For this review, take the finished solid that the model builds, in its own axes (mm). A direction names the side the tool comes from. Round coordinates to 2 decimals unless told otherwise and drop trailing zeros. Loops run counter-clockwise (first coordinate to the right, second up) from the corner with the lowest first, then second, coordinate; pieces in that order, holes last. Notation, with made-up numbers: M -31.75,6.25 L 12.25,6.25 A13 ccw 12.25,24.25 Z; hole C 25,65.25 d7. An arc over 180 degrees is marked long. One line per question, with ' | ' between items. Start each with the question number.
1) For pin 1 Ø3.5 at (x, z) = (49, 57.5) entering from +Y; pin 2 Ø0.9 at (x, z) = (-49, 57.5) entering from -Y; pin 3 Ø0.9 at (x, y) = (49, -1) entering from +Z, all flat-tipped, find the tip position at first contact; note any pin that passes through.
2) Mouldability with a two-part tool opening along X and no side actions: class faces 5 (the face through (-49, 29, 30)), 6 (the face through (47, 0, 30)), 7 (the face through (-48, -5, 58)) as pulls with the +X half, pulls with the -X half, needs draft (parallel to the pull), parting line crosses it, or undercut.
3) We need section D-D (z = 47.5). Give the boundary of the cut face in (x, y), and give its area (3 significant figures).
4) We need section B-B (y = 2). Give the boundary of the cut face in (x, z).
5) For probe 1 along Y at (x, z) = (-37, 19); probe 2 along X at (y, z) = (-3, 14.5); probe 3 along X at (y, z) = (26.5, 24), list the stretches that pass through material, from the lowest coordinate up. Write a range as from..to.
6) For faces 1 (the face through (-3, 30, 0)), 2 (the face through (-1, 28, 30)), 3 (the face through (49, 5, 58)), 4 (the face through (25, -30, 26)), list the 3-axis set-ups (+Z, -Z, +X, -X, +Y, -Y) from which the entire face can be reached by the end or side of a thin tool; tool diameter is ignored.
7) We need section A-A (x = -33.5). Give the boundary of the cut face in (y, z), and give its area (3 significant figures).
8) We need section C-C (x = 25). Give the boundary of the cut face in (y, z), and give its area (3 significant figures).
```python
from build123d import *

# Parameters (mm, degrees)
EXTRUDE_1_DEPTH          = 60
EXTRUDE_2_DEPTH          = 60
SKETCH_4_R               = 1.4
CUT_EXTRUDE_1_DEPTH      = 60
MIRROR_2_COPY_1_DEPTH    = 60
MIRROR_2_COPY_2_SKETCH_R = 1.4
MIRROR_2_COPY_2_DEPTH    = 60
SKETCH_7_R               = 6
CUT_EXTRUDE_3_DEPTH      = 10
SKETCH_8_W               = 4
SKETCH_8_H               = 10
CUT_EXTRUDE_4_DEPTH      = 100


with BuildPart() as part:
    # 草图1 → 凸台-拉伸1 (new body)
    with BuildSketch(Plane.XY):
        with BuildLine():
            Line((-45, 31), (45, 31))
            ThreePointArc((45, 31), (48.535533906, 29.535533906), (50, 26))
            Line((50, 26), (50, -26))
            ThreePointArc((50, -26), (48.535533906, -29.535533906), (45, -31))
            Line((45, -31), (-45, -31))
            ThreePointArc((-45, -31), (-48.535533906, -29.535533906), (-50, -26))
            Line((-50, -26), (-50, 26))
            ThreePointArc((-50, 26), (-48.535533906, 29.535533906), (-45, 31))
        make_face()
        with BuildLine():
            Line((-42, 28), (42, 28))
            ThreePointArc((42, 28), (45.535533906, 26.535533906), (47, 23))
            Line((47, 23), (47, -23))
            ThreePointArc((47, -23), (45.535533906, -26.535533906), (42, -28))
            Line((42, -28), (-42, -28))
            ThreePointArc((-42, -28), (-45.535533906, -26.535533906), (-47, -23))
            Line((-47, -23), (-47, 23))
            ThreePointArc((-47, 23), (-45.535533906, 26.535533906), (-42, 28))
        make_face(mode=Mode.SUBTRACT)
    extrude(amount=EXTRUDE_1_DEPTH)

    # 草图3 → 凸台-拉伸2 (add)
    with BuildSketch(Plane.XY.offset(60)):
        Polygon((-47, 28), (-47, 21), (-40, 28), align=None)
    extrude_2 = extrude(amount=-EXTRUDE_2_DEPTH)

    # 草图4 → 切除-拉伸1 (cut)
    with BuildSketch(Plane.XY.offset(60)):
        with Locations((-46, 27)):
            Circle(SKETCH_4_R)
    cut_extrude_1 = extrude(amount=-CUT_EXTRUDE_1_DEPTH, mode=Mode.SUBTRACT)

    # 镜向1: 凸台-拉伸2, 切除-拉伸1 across plane
    add(extrude_2.mirror(Plane(origin=(0, 0, 0), x_dir=(0, 0, 1), z_dir=(1, 0, 0))))
    add(cut_extrude_1.mirror(Plane(origin=(0, 0, 0), x_dir=(0, 0, 1), z_dir=(1, 0, 0))), mode=Mode.SUBTRACT)

    # 镜向2: 凸台-拉伸2, 切除-拉伸1 across plane
    add(extrude_2.mirror(Plane.ZX))
    add(cut_extrude_1.mirror(Plane.ZX), mode=Mode.SUBTRACT)

    # 镜向2 copy 1 sketch → 镜向2 copy 1 (add)
    with BuildSketch(Plane(origin=(0, 0, 60), x_dir=(-1, 0, 0), z_dir=(0, 0, 1))):
        Polygon((-47, 28), (-47, 21), (-40, 28), align=None)
    extrude(amount=-MIRROR_2_COPY_1_DEPTH)

    # 镜向2 copy 2 sketch → 镜向2 copy 2 (cut)
    with BuildSketch(Plane(origin=(0, 0, 60), x_dir=(-1, 0, 0), z_dir=(0, 0, 1))):
        with Locations((-46, 27)):
            Circle(MIRROR_2_COPY_2_SKETCH_R)
    extrude(amount=-MIRROR_2_COPY_2_DEPTH, mode=Mode.SUBTRACT)

    # 草图7 → 切除-拉伸3 (cut)
    with BuildSketch(Plane.XZ.offset(31)):
        with Locations(Location((-25, 20, 0), (0, 0, 270))):
            Circle(SKETCH_7_R)
        with Locations(Location((25, 20, 0), (0, 0, 270))):
            Circle(SKETCH_7_R)
    extrude(amount=-CUT_EXTRUDE_3_DEPTH, mode=Mode.SUBTRACT)

    # 草图8 → 切除-拉伸4 (cut)
    with BuildSketch(Plane(origin=(50, 0, 0), x_dir=(0, 0, -1), z_dir=(1, 0, 0))):
        with Locations((-58, 0)):
            Rectangle(SKETCH_8_W, SKETCH_8_H)
    extrude(amount=-CUT_EXTRUDE_4_DEPTH, mode=Mode.SUBTRACT)


solid = part.part
```
Answers below:
1) pin 1: y = 30.47 | pin 2: y = -29.52 | pin 3: z = 56
2) face 5: pulls with the -X half | face 6: undercut | face 7: needs draft
3) outline: M -50,-26 A5 ccw -45,-31 L 45,-31 A5 ccw 50,-26 L 50,26 A5 ccw 45,31 L -45,31 A5 ccw -50,26 Z; hole C -46,-27 d2.8; hole C -46,27 d2.8; hole M -47,-21 L -40,-28 L 40,-28 L 47,-21 L 47,21 L 40,28 L -40,28 L -47,21 Z; hole C 46,-27 d2.8; hole C 46,27 d2.8 | area: 988 mm^2
4) outline: M -50,0 L -47,0 L -47,56 L -50,56 Z; M 47,0 L 50,0 L 50,56 L 47,56 Z
5) probe 1: -31..-28, 28..31 | probe 2: -50..-47, 47..50 | probe 3: -49.97..-47.31, -44.69..-41.5, 41.5..44.69, 47.31..49.97
6) face 1: -Z, +X, -X, +Y, -Y | face 2: +Z, -Z | face 3: +Z, +X, -X | face 4: -Y
7) outline: M -31,0 L -28,0 L -28,60 L -31,60 Z; M 28,0 L 31,0 L 31,60 L 28,60 Z | area: 360 mm^2
8) outline: M -31,0 L -28,0 L -28,14 L -31,14 Z; M -31,26 L -28,26 L -28,60 L -31,60 Z; M 28,0 L 31,0 L 31,60 L 28,60 Z | area: 324 mm^2
